```python
from build123d import *

# Parameters (mm, degrees)
EXTRUDE_1_DEPTH              = 120
SKETCH_2_W                   = 48.5
SKETCH_2_H                   = 20
EXTRUDE_2_DEPTH              = 25
HOLE_WIZARD_M4_1_D           = 3.3
HOLE_WIZARD_M4_1_ON_FACE_2_D = 3.3
CUT_EXTRUDE_1_REACH          = 161.463


with BuildPart() as part:
    # 草图1 → 凸台-拉伸1 (new body)
    with BuildSketch(Plane(origin=(0, 51.506568262, -7630.363691544), x_dir=(1, 0, 0), z_dir=(0, -0.006750057654754126, 0.9999772181013213))):
        Polygon((28.350451638, 9.735119508), (36.350451638, 9.735119508), (36.350451638, 24.735119508), (16.350451638, 24.735119508), (16.350451638, 14.735119508), (28.350451638, 14.735119508), align=None)
        Polygon((36.350451638, 24.735119508), (36.350451638, 9.735119508), (44.350451638, 9.735119508), (44.350451638, 14.735119508), (56.350451638, 14.735119508), (56.350451638, 24.735119508), (47.100400838, 24.735119508), (47.100400838, 22.735119508), (47.100400838, 17.735119508), (41.100400838, 17.735119508), (41.100400838, 22.735119508), (41.100400838, 24.735119508), align=None)
    extrude(amount=-EXTRUDE_1_DEPTH)

    # 草图2 → 凸台-拉伸2 (add)
    with BuildSketch(Plane(origin=(0, 51.506568262, -7630.363691544), x_dir=(1, 0, 0), z_dir=(0, -0.00675005765475416, 0.9999772181013213))):
        with Locations((36.350451638, 17.235119507)):
            Rectangle(SKETCH_2_W, SKETCH_2_H)
    extrude(amount=EXTRUDE_2_DEPTH)

    # M4 螺纹孔1 (through all)
    with Locations(Plane(origin=(47.850451638, 78.639816437, -7615.180194646), x_dir=(0, -0.006750057655, 0.999977218101), z_dir=(0, 0.999977218101, 0.006750057655))):
        with Locations((0, 0)):
            Hole(HOLE_WIZARD_M4_1_D / 2)

    # M4 螺纹孔1 on face 2 (through all)
    with Locations(Plane(origin=(24.850451638, 78.639816437, -7615.180194646), x_dir=(0, -0.006750001475, 0.999977218481), z_dir=(0, 0.999977218481, 0.006750001475))):
        with Locations((0, 0)):
            Hole(HOLE_WIZARD_M4_1_ON_FACE_2_D / 2)

    # 草图5 → 切除-拉伸1 (cut, up to next)
    with BuildSketch(Plane(origin=(0, 51.337816821, -7605.364261092), x_dir=(1, 0, 0), z_dir=(0, -0.0067500576547363505, 0.9999772181013213)), mode=Mode.PRIVATE) as cut_extrude_1_sk1:
        Polygon((12.100451638, 17.235119508), (22.100451638, 7.235119508), (12.100451638, 7.235119508), align=None)
    cut_extrude_1_tool1 = extrude(cut_extrude_1_sk1.sketch, amount=-CUT_EXTRUDE_1_REACH, mode=Mode.PRIVATE) & part.part
    # 草图5 → 切除-拉伸1 (cut, up to next)
    with BuildSketch(Plane(origin=(0, 51.337816821, -7605.364261092), x_dir=(1, 0, 0), z_dir=(0, -0.0067500576547363505, 0.9999772181013213)), mode=Mode.PRIVATE) as cut_extrude_1_sk2:
        Polygon((60.600451638, 17.235119508), (50.600451638, 7.235119508), (60.600451638, 7.235119508), align=None)
    cut_extrude_1_tool2 = extrude(cut_extrude_1_sk2.sketch, amount=-CUT_EXTRUDE_1_REACH, mode=Mode.PRIVATE) & part.part
    add(cut_extrude_1_tool1.solids().sort_by_distance((15.433785, 61.906029, -7605.292923))[0], mode=Mode.SUBTRACT)
    add(cut_extrude_1_tool2.solids().sort_by_distance((57.267118, 61.906029, -7605.292923))[0], mode=Mode.SUBTRACT)


solid = part.part
```
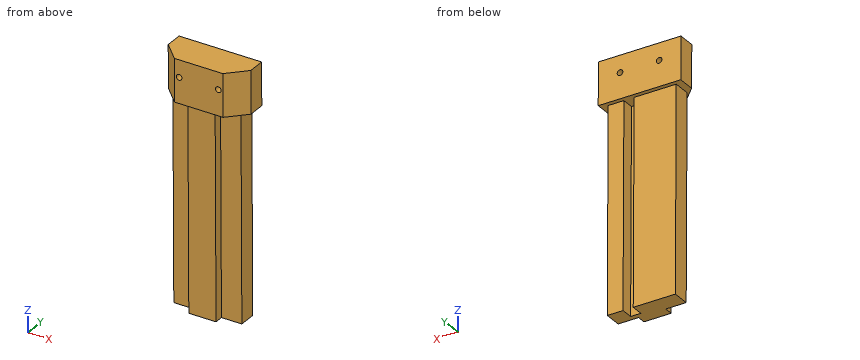
For this review, take the finished solid that the model builds, in its own axes (mm). Coordinates: 2 decimals unless noted, no trailing zeros. Write each loop counter-clockwise with the first axis right and the second up, starting at its lowest first coordinate (ties: lowest second). Pieces come first, ordered by that corner, then holes.
(1) For pin 1 Ø4 at (x, z) = (29, -7682.5) entering from -Y; pin 2 Ø2.5 at (y, z) = (71.5, -7715.5) entering from +X; pin 3 Ø6 at (x, z) = (53, -7651) entering from -Y, all flat-tipped, find the tip position at first contact; note any pin that passes through.
(2) Wall thickness on probe 1 along X at (y, z) = (73.5, -7689.5); probe 2 along X at (y, z) = (76.5, -7616); probe 3 along X at (y, z) = (63.5, -7743): over which ranges is each line inside the solid? List them lowest first.
(3) Add section D-D on x = 54. Give the boundary of the cut face in (y, z), then the cut area to 3 significant figures.
(4) Add section B-B on z = -7663. Give the boundary of the cut face in (x, y), then the cut area to 3 significant figures.
(5) Add section C-C on y = 75. Count the separate pieces of the cut face and the enclosed holes in it, then the cut area to 3 significant figures.
(6) Add section A-A on x = 32.5. Give the boundary of the cut face in (y, z), then the cut area to 3 significant figures.
Answer sheet:
1. pin 1: stops at y = 61.58
1. pin 2: stops at x = 56.35
1. pin 3: stops at y = 66.36
2. probe 1: x = 16.35 to 41.1, 47.1 to 56.35
2. probe 2: x = 12.1 to 23.41, 26.29 to 46.41, 49.29 to 60.6
2. probe 3: x = 28.35 to 44.35
3. outline: (61.97, -7605.29) - (62.14, -7630.29) - (66.24, -7630.26) - (67.05, -7750.26) - (77.05, -7750.19) - (76.24, -7630.2) - (78.74, -7630.18) - (78.57, -7605.18) - close
3. area: 1,620 mm2
4. outline: (16.35, 66.46) - (28.35, 66.46) - (28.35, 61.46) - (44.35, 61.46) - (44.35, 66.46) - (56.35, 66.46) - (56.35, 76.46) - (47.1, 76.46) - (47.1, 69.46) - (41.1, 69.46) - (41.1, 76.46) - (16.35, 76.46) - close
4. area: 438 mm2
5. separate pieces: 1
5. enclosed holes: 2
5. area: 5,280 mm2
6. outline: (58.57, -7605.32) - (58.74, -7630.31) - (61.24, -7630.3) - (62.05, -7750.3) - (77.05, -7750.19) - (76.24, -7630.2) - (78.74, -7630.18) - (78.57, -7605.18) - close
6. area: 2,300 mm2
